from build123d import *

# Parameters (mm, degrees)
SKETCH_1_R      = 8
EXTRUDE_1_DEPTH = 3
SKETCH_2_R      = 4
EXTRUDE_2_DEPTH = 30
CHAMFER_1_SIZE  = 0.6


with BuildPart() as part:
    # Эскиз1 → Бобышка-Вытянуть1 (new body)
    with BuildSketch(Plane(origin=(0, 0, 0), x_dir=(1, 0, 0), z_dir=(0, 1, 0))):
        with Locations(Location((0, 0, 0), (0, 0, 270))):
            Circle(SKETCH_1_R)
    extrude(amount=EXTRUDE_1_DEPTH)

    # Эскиз2 → Бобышка-Вытянуть2 (add)
    with BuildSketch(Plane(origin=(0, 3, 0), x_dir=(1, 0, 0), z_dir=(0, 1, 0))):
        with Locations(Location((0, 0, 0), (0, 0, 270))):
            Circle(SKETCH_2_R)
    extrude(amount=EXTRUDE_2_DEPTH)

    # Эскиз3 → Вырез-Повернуть1 (revolve, cut)
    with BuildSketch(Plane(origin=(0, 0, 0), x_dir=(0, 0, -1), z_dir=(1, 0, 0)), mode=Mode.PRIVATE) as cut_revolve_1_sk:
        Polygon((-8, 0), (0, 2.143593539), (0, 0), align=None)
    revolve(cut_revolve_1_sk.sketch.rotate(Axis((0, 2.143593539, 0), (0, -1, 0)), 180), axis=Axis((0, 2.143593539, 0), (0, -1, 0)), mode=Mode.SUBTRACT)

    # Фаска1
    chamfer_1_edges = [part.edges().sort_by_distance(p)[0] for p in [
        (0, 33, -4),
    ]]
    chamfer(chamfer_1_edges, length=CHAMFER_1_SIZE)


solid = part.part
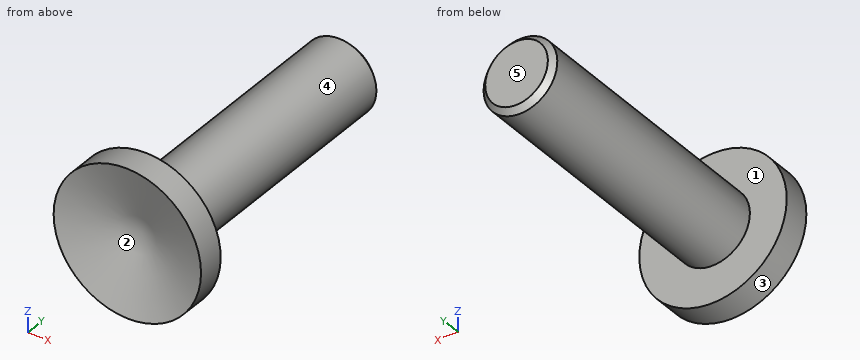
CAD build for the part. Positions are in the model's coordinates, mm. Face numbers are marked on the shaded views. A direction names the side the tool comes from. Coordinates: 2 decimals unless noted, no trailing zeros. Loops run counter-clockwise (first coordinate to the right, second up) from the corner with the lowest first, then second, coordinate; pieces in that order, holes last. Notation, with made-up numbers: (-39.5, -3) - (-13.5, -3) arc R22 ccw to (-13.5, 8) - close; hole circle Ø8 at (-37.75, 82.25). An arc over 180 degrees is marked (long way). Write item = value, one per line. Start each with the question number.
Q1. Flat gauge pins, fed straight in: pin 1 Ø1 at (x, z) = (3.5, -2.5) entering from -Y; pin 2 Ø6 at (x, y) = (1.5, 23.5) entering from -Z; pin 3 Ø4 at (x, z) = (-5.5, -1.5) entering from -Y; pin 4 Ø6 at (x, z) = (4, 1.5) entering from +Y. Where does each tip first touch, or does it go through?
Q2. Cut at A-A, the plane y = 29.5. List the corners of the cut face in (x, z).
Q3. Pull direction X, two halves, no side cores. Call the marked faces 1, 2 and 3: pulls with the +X half, pulls with the -X half, needs draft (parallel to the pull), parting line crosses it, or undercut.
Q4. Which spindle directions (+Z, -Z, +X, -X, +Y, -Y) get a long thin tool onto all of the face, cutting with end or side? Do the marked faces 4 and 5. Say none if no direction does.
Q5. Drill centre lines: L1, parallel to Z at x = -2.25, y = 17; L2, parallel to Y at x = 1.5, z = 7.75; L3, parallel to Y at x = -4.25, z = 3.5. Where is each one in solid material? Low to high.
Computed:
q1.pin_1 = 0.86
q1.pin_2 = -4
q1.pin_3 = 0.08
q1.pin_4 = 33
q2.outline = circle Ø8 at (0, 0)
q3.face_1 = needs draft
q3.face_2 = undercut
q3.face_3 = parting line crosses it
q4.face_4 = +Y
q4.face_5 = +Z, -Z, +X, -X, +Y
q5.L1 = -3.31 to 3.31
q5.L2 = 0.03 to 3
q5.L3 = 0.67 to 3
